Geometry check sheet. Reference: the model listing, model coordinates, mm. Face numbers are marked on the shaded views. A direction names the side the tool comes from. Give positions to 0.01 mm unless a question says otherwise; leave off trailing zeros. Loops run counter-clockwise (first coordinate to the right, second up) from the corner with the lowest first, then second, coordinate; pieces in that order, holes last. Notation, with made-up numbers: (-14, 38.5) -> (18, 38.5) arc R29 ccw to (18, 63.5) -> close; hole circle Ø3 at (-22, 15.5). An arc over 180 degrees is marked (long way). Answer as a JSON object with one key per item and string values.
from build123d import *

# Parameters (mm, degrees)
F1_DEPTH = 56
F2_R     = 1
F3_R     = 6
F5_DEPTH = 99.1


with BuildPart() as f1:
    # F0 (on Front) → F1 (new body)
    with BuildSketch(Plane.XZ):
        Polygon((42.5, 17.5), (-42.5, 17.5), (-42.5, -17.5), (-37.5, -17.5), (37.5, -17.5), (42.5, -17.5), align=None)
        Polygon((-37.5, -17.5), (-42.5, -17.5), (-42.5, -22.5), align=None)
        Polygon((42.5, -22.5), (42.5, -17.5), (37.5, -17.5), align=None)
    extrude(amount=F1_DEPTH)

    # F2
    f2_edges = [f1.edges().sort_by_distance(p)[0] for p in [
        (-42.5, -28, -22.5),
        (42.5, -28, -22.5),
    ]]
    fillet(f2_edges, radius=F2_R)

    # F3
    f3_edges = [f1.edges().sort_by_distance(p)[0] for p in [
        (-42.5, -28, 17.5),
        (42.5, -28, 17.5),
    ]]
    fillet(f3_edges, radius=F3_R)

    # F4 (on face) → F5 (cut)
    with BuildSketch(Plane.XZ.offset(56)):
        with BuildLine():
            Line((-37.997056, -16.3), (37.997056, -16.3))
            Line((37.997056, -16.3), (41.3, -19.602944))
            Line((41.3, -19.602944), (41.3, 11.5))
            ThreePointArc((41.3, 11.5), (39.894113, 14.894113), (36.5, 16.3))
            Line((36.5, 16.3), (-36.5, 16.3))
            ThreePointArc((-36.5, 16.3), (-39.894113, 14.894113), (-41.3, 11.5))
            Line((-41.3, 11.5), (-41.3, -19.602944))
            Line((-41.3, -19.602944), (-37.997056, -16.3))
        make_face()
    extrude(amount=-F5_DEPTH, mode=Mode.SUBTRACT)


solid = f1.part
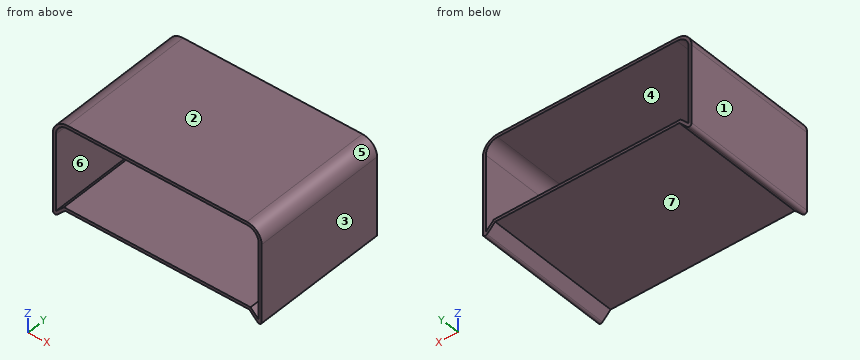
1) Section check A-A on y = -24. Record the cut outline in (x, z).
Geometry check:
{"outline": "(-42.5, -20.09) arc R1 ccw to (-40.79, -20.79) -> (-37.5, -17.5) -> (37.5, -17.5) -> (40.79, -20.79) arc R1 ccw to (42.5, -20.09) -> (42.5, 11.5) arc R6 ccw to (36.5, 17.5) -> (-36.5, 17.5) arc R6 ccw to (-42.5, 11.5) -> close; hole (-41.3, -19.6) -> (-38, -16.3) -> (38, -16.3) -> (41.3, -19.6) -> (41.3, 11.5) arc R4.8 ccw to (36.5, 16.3) -> (-36.5, 16.3) arc R4.8 ccw to (-41.3, 11.5) -> close"}
2) Draft check along X on the marked faces 1, 2, 3 and 4. Enter one of: pulls with the +X half, pulls with the -X half, needs draft (parallel to the pull), parting line crosses it, or undercut.
Geometry check:
{"face 1": "pulls with the -X half", "face 2": "needs draft", "face 3": "pulls with the +X half", "face 4": "undercut"}
3) Section check C-C on x = -34. Record the cut outline in (y, z).
Geometry check:
{"outline": "(-56, -17.5) -> (0, -17.5) -> (0, -16.3) -> (-56, -16.3) -> close; (-56, 16.3) -> (0, 16.3) -> (0, 17.5) -> (-56, 17.5) -> close"}
4) Material ranges on line 1 along Z through (x, y) = (-24, -10); line 2 along X through (y, z) = (-44.5, -6); line 3 along X through (y, z) = (-14, -18), recorded low to high. Write a range as from..to.
Geometry check:
{"line 1": "z = -17.5..-16.3, 16.3..17.5", "line 2": "x = -42.5..-41.3, 41.3..42.5", "line 3": "x = -42.5..-41.3, -39.7..-38, 38..39.7, 41.3..42.5"}
5) Depth check by flat-ended pin: P1, Ø8, axis at x = -6.5, y = -42.5, coming from the -Z side; P2, Ø1.5, axis at x = 32.5, z = -16.5, coming from the +Y side. Enter the tip coordinate at first touch or a pass-through.
Geometry check:
{"P1": "stops at z = -17.5", "P2": "stops at y = 0"}
6) Section check B-B on z = -5. Record the cut outline in (x, y).
Geometry check:
{"outline": "(-42.5, -56) -> (-41.3, -56) -> (-41.3, 0) -> (-42.5, 0) -> close; (41.3, -56) -> (42.5, -56) -> (42.5, 0) -> (41.3, 0) -> close"}
7) Tool access check on the marked faces 5, 6 and 7. Record the directions out of +Z, -Z, +X, -X, +Y, -Y that give a thin tool (end or side, any length) a straight path to the whole face; none if there is none.
Geometry check:
{"face 5": "+Z, +X, +Y, -Y", "face 6": "+Y, -Y", "face 7": "-Z, +Y, -Y"}
